```python
from build123d import *

# Parameters (mm, degrees)
SKETCH1_W           = 60
SKETCH1_H           = 30
BOSS_EXTRUDE1_DEPTH = 5
BOSS_EXTRUDE4_DEPTH = 32
SKETCH7_W           = 40.9
SKETCH7_H           = 22.76
BOSS_EXTRUDE5_DEPTH = 12
SKETCH9_R           = 2
CUT_EXTRUDE2_DEPTH  = 5
SKETCH10_R          = 2
CUT_EXTRUDE3_DEPTH  = 4


with BuildPart() as part:
    # Sketch1 → Boss-Extrude1 (new body)
    with BuildSketch(Plane(origin=(0, 0, 0), x_dir=(1, 0, 0), z_dir=(0, 1, 0))):
        Rectangle(SKETCH1_W, SKETCH1_H)
    extrude(amount=BOSS_EXTRUDE1_DEPTH)

    # Sketch6 → Boss-Extrude4 (add)
    with BuildSketch(Plane(origin=(0, 5, 0), x_dir=(1, 0, 0), z_dir=(0, 1, 0))):
        Polygon((-20.45, 15), (-25.45, 15), (-25.45, -2.76), (-30, -2.76), (-30, -7.76), (-20.45, -7.76), align=None)
        Polygon((30, -2.76), (30, -7.76), (20.45, -7.76), (20.45, 15), (25.45, 15), (25.45, -2.76), align=None)
    extrude(amount=BOSS_EXTRUDE4_DEPTH)

    # Sketch7 → Boss-Extrude5 (add)
    with BuildSketch(Plane(origin=(0, 5, 0), x_dir=(1, 0, 0), z_dir=(0, 1, 0))):
        with Locations((0, 3.62)):
            Rectangle(SKETCH7_W, SKETCH7_H)
    extrude(amount=BOSS_EXTRUDE5_DEPTH)

    # Sketch9 → Cut-Extrude2 (cut)
    with BuildSketch(Plane(origin=(0, 5, 0), x_dir=(1, 0, 0), z_dir=(0, 1, 0))):
        with Locations(Location((-25, -11.5, 0), (0, 0, 270))):
            Circle(SKETCH9_R)
        with Locations(Location((25, -11.5, 0), (0, 0, 270))):
            Circle(SKETCH9_R)
    extrude(amount=-CUT_EXTRUDE2_DEPTH, mode=Mode.SUBTRACT)

    # Sketch10 → Cut-Extrude3 (cut)
    with BuildSketch(Plane.XY.offset(7.76)):
        with Locations((-24.3, 32)):
            Circle(SKETCH10_R)
        with Locations((-24.3, 22)):
            Circle(SKETCH10_R)
        with Locations(Location((24.3, 22, 0), (0, 0, 180))):
            Circle(SKETCH10_R)
        with Locations(Location((24.3, 32, 0), (0, 0, 180))):
            Circle(SKETCH10_R)
    extrude(amount=-CUT_EXTRUDE3_DEPTH, mode=Mode.SUBTRACT)


solid = part.part
```
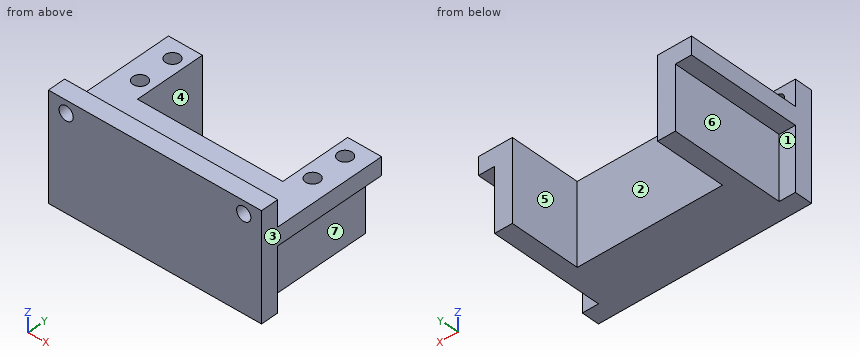
The model under review builds one solid part; all positions refer to its coordinate system, in mm. Face numbers are marked on the shaded views. A direction names the side the tool comes from. Coordinates: 2 decimals unless noted, no trailing zeros. Write each loop counter-clockwise with the first axis right and the second up, starting at its lowest first coordinate (ties: lowest second). Pieces come first, ordered by that corner, then holes. Notation, with made-up numbers: (52, 29.5) -> (80, 29.5) arc R19 ccw to (80, 64.5) -> close; hole circle Ø5 at (-18, 48). An arc over 180 degrees is marked (long way). One line per item, written item: value. Start each with the question number.
Q1. Clearance check with flat-ended pins moving along their axes: P1, Ø1, axis at x = -5, z = -11, coming from the +Y side; P2, Ø4, axis at y = 30, z = 0.5, coming from the +X side; P3, Ø3.5, axis at x = 6.5, z = 12, coming from the +Y side. State where each tip first meets the part, or that it passes through.
Q2. Add section C-C, the plane z = 11.5. Give the boundary of the cut face in (x, y).
Q3. For the marked faces 5, 6 and 7, list the 3-axis set-ups (+Z, -Z, +X, -X, +Y, -Y) from which the entire face can be reached by the end or side of a thin tool; tool diameter is ignored.
Q4. Add section B-B, the plane y = 13. Give the boundary of the cut face in (x, z), then the cut area to 3 significant figures.
Q5. To check wall thickness, follow probe 1 along Y at (x, z) = (24.3, 6.3); probe 2 along X at (y, z) = (3.35, 11.5); probe 3 along X at (y, z) = (19, -6.5). State the ranges of each line that lie inside material, in increasing order.
Q6. Add section A-A, the plane z = 5.75. Give the boundary of the cut face in (x, y), then the cut area to 3 significant figures.
Q7. The part is to be moulded in two halves that separate along X. For the marked faces 1, 2, 3 and 4, say which applies: +X half, -X half, draft (parallel to the pull), parting line (faces both ways), or undercut.
Q8. Add section D-D, the plane y = 22. Give the boundary of the cut face in (x, z).
Response:
1. P1: y = 17
1. P2: x = 25.45
1. P3: y = 5
2. outline: (-30, 0) -> (-27, 0) -> (-27, 5) -> (-30, 5) -> close; (-23, 0) -> (23, 0) -> (23, 5) -> (-23, 5) -> close; (27, 0) -> (30, 0) -> (30, 5) -> (27, 5) -> close
3. face 5: +Z, -Z, +Y
3. face 6: -Z, -X, +Y
3. face 7: -Z, +X, +Y
4. outline: (-30, 2.76) -> (-25.45, 2.76) -> (-25.45, -15) -> (25.45, -15) -> (25.45, 2.76) -> (30, 2.76) -> (30, 7.76) -> (-30, 7.76) -> close
4. area: 1,200 mm²
5. probe 1: 0 to 20, 24 to 30, 34 to 37
5. probe 2: -30 to -27, -23 to 23, 27 to 30
5. probe 3: -25.45 to -20.45, 20.45 to 25.45
6. outline: (-30, 0) -> (30, 0) -> (30, 37) -> (20.45, 37) -> (20.45, 17) -> (-20.45, 17) -> (-20.45, 37) -> (-30, 37) -> close; hole circle Ø4 at (-24.3, 22); hole circle Ø4 at (-24.3, 32); hole circle Ø4 at (24.3, 22); hole circle Ø4 at (24.3, 32)
6. area: 1,350 mm²
7. face 1: draft
7. face 2: undercut
7. face 3: +X half
7. face 4: undercut
8. outline: (-30, 2.76) -> (-25.45, 2.76) -> (-25.45, -15) -> (-20.45, -15) -> (-20.45, 7.76) -> (-22.3, 7.76) -> (-22.3, 3.76) -> (-26.3, 3.76) -> (-26.3, 7.76) -> (-30, 7.76) -> close; (20.45, -15) -> (25.45, -15) -> (25.45, 2.76) -> (30, 2.76) -> (30, 7.76) -> (26.3, 7.76) -> (26.3, 3.76) -> (22.3, 3.76) -> (22.3, 7.76) -> (20.45, 7.76) -> close
